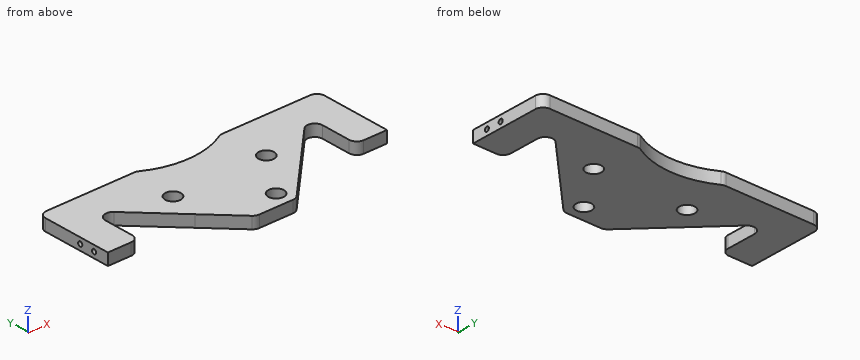
```python
from build123d import *

# Parameters (mm, degrees)
BOSS_EXTRUDE1_DEPTH             = 9.525
F_1_2_0_5_DIAMETER_HOLE1_D      = 12.7
SKETCH7_R                       = 66.675
CUT_EXTRUDE1_DEPTH              = 169.325445566
CUT_EXTRUDE2_DEPTH              = 169.325445566
FILLET1_R                       = 6.35
F_10_24_TAPPED_HOLE1_AT_2_COUNT = 2
F_10_24_TAPPED_HOLE1_AT_2_PITCH = 12.7


with BuildPart() as part:
    # Sketch2 → Boss-Extrude1 (new body)
    with BuildSketch(Plane.XY):
        Polygon((-16.500012242, 33.286517476), (16.500012242, 33.286517476), (42.913494767, 59.7), (114.3, 59.7), (114.3, 123.2), (-114.3, 123.2), (-114.3, 59.7), (-42.913494767, 59.7), align=None)
    extrude(amount=BOSS_EXTRUDE1_DEPTH)

    # 1/2 (0.5) Diameter Hole1 (through all)
    with Locations(Plane.XY.offset(9.525)):
        with Locations((-38.227, 85.227), (38.227, 85.227), (11.2395, 45.986517476)):
            Hole(F_1_2_0_5_DIAMETER_HOLE1_D / 2)

    # Sketch7 → Cut-Extrude1 (cut, through all)
    with BuildSketch(Plane(origin=(0, 0, 0), x_dir=(-1, 0, 0), z_dir=(0, 0, -1))):
        with Locations((0, 180.35)):
            Circle(SKETCH7_R)
    extrude(amount=-CUT_EXTRUDE1_DEPTH, mode=Mode.SUBTRACT)

    # Sketch13 → Cut-Extrude2 (cut, through all)
    with BuildSketch(Plane(origin=(0, 0, 0), x_dir=(-1, 0, 0), z_dir=(0, 0, -1))):
        Polygon((42.913494767, 59.7), (88.9, 105.686505233), (88.9, 59.7), align=None)
        Polygon((-42.913494767, 59.7), (-88.9, 105.686505233), (-88.9, 59.7), align=None)
    extrude(amount=-CUT_EXTRUDE2_DEPTH, mode=Mode.SUBTRACT)

    # Fillet1
    fillet1_edges = [part.edges().sort_by_distance(p)[0] for p in [
        (-114.3, 123.2, 4.7625),
        (114.3, 123.2, 4.7625),
        (16.500012242, 33.286517476, 4.7625),
        (-16.500012242, 33.286517476, 4.7625),
        (-34.342875899, 123.2, 4.7625),
        (34.342875899, 123.2, 4.7625),
        (-88.9, 59.7, 4.7625),
        (-88.9, 105.686505233, 4.7625),
        (88.9, 59.7, 4.7625),
        (88.9, 105.686505233, 4.7625),
    ]]
    fillet(fillet1_edges, radius=FILLET1_R)

    # Sketch12 → #10-24 Tapped Hole1 (revolve, cut)
    with BuildSketch(Plane(origin=(-114.3, 85.1, 4.7625), x_dir=(0, 0, 1), z_dir=(0, 1, 0))):
        Polygon((0, 0), (0, 16.088724014), (1.89865, 14.9479), (1.89865, 0), align=None)
    f_10_24_tapped_hole1 = revolve(axis=Axis((-120.65, 85.1, 4.7625), (1, 0, 0)), mode=Mode.SUBTRACT)

    # #10-24 Tapped Hole1 at 2: #10-24 Tapped Hole1 ×2
    with Locations(*[(0, -i * F_10_24_TAPPED_HOLE1_AT_2_PITCH, 0) for i in range(1, F_10_24_TAPPED_HOLE1_AT_2_COUNT)]):
        add(f_10_24_tapped_hole1, mode=Mode.SUBTRACT)

    # Mirror1: #10-24 Tapped Hole1 across plane
    add(f_10_24_tapped_hole1.mirror(Plane(origin=(0, 0, 0), x_dir=(0, 0, 1), z_dir=(1, 0, 0))), mode=Mode.SUBTRACT)

    # Mirror1 copy 1 sketch → Mirror1 copy 1 (revolve, cut)
    with BuildSketch(Plane(origin=(114.3, 72.4, 4.7625), x_dir=(0, 0, 1), z_dir=(0, 1, 0))):
        Polygon((0, 0), (0, -16.088724014), (1.89865, -14.9479), (1.89865, 0), align=None)
    revolve(axis=Axis((120.65, 72.4, 4.7625), (1, 0, 0)), mode=Mode.SUBTRACT)


solid = part.part
```
CAD build for the part. Positions are in the model's coordinates, mm. Round coordinates to 2 decimals unless told otherwise and drop trailing zeros. Order: outer loops, then holes, each group sorted by start corner. A loop starts at its lowest first (then second) coordinate and runs counter-clockwise, first axis right, second up. Notation, with made-up numbers: (18.5, 28) - (36.5, 28) arc R21 ccw to (36.5, 56) - close; hole circle Ø4 at (29.25, 53.5). An arc over 180 degrees is marked (long way). Use CSV: the item, a comma, the result in double quotes. Start each with the question number.
1) Saw through at A-A (y = 81). List the corners of the cut face in (x, z) (1 decimal), and give its area (3 significant figures).
2) Pin check, flat tips, straight feed: pin 1 Ø3 at (x, z) = (107, 4.5) entering from -Y; pin 2 Ø4 at (x, z) = (-52, 1.5) entering from -Y. Stop position of each tip, or through.
3) Saw through at B-B (x = -91.5). List the corners of the cut face in (y, z) (3 decimals), and give its area (3 significant figures).
4) Wall check: L1, parallel to Z at x = -107, y = 72.4 (3 decimals); L2, parallel to Y at x = 96.5, z = 0.75; L3, parallel to X at y = 86, z = 2. Give the ranges that are in metal, low to high. Write a range as [from, to].
5) Saw through at C-C (x = -66). List the corners of the cut face in (y, z) (1 decimal), and give its area (3 significant figures).
Values follow:
1,outline,"(-114.3, 0) - (-88.9, 0) - (-88.9, 9.5) - (-114.3, 9.5) - close; (-64.2, 0) - (-43, 0) - (-43, 9.5) - (-64.2, 9.5) - close; (-33.5, 0) - (33.5, 0) - (33.5, 9.5) - (-33.5, 9.5) - close; (43, 0) - (64.2, 0) - (64.2, 9.5) - (43, 9.5) - close; (88.9, 0) - (114.3, 0) - (114.3, 9.5) - (88.9, 9.5) - close"
1,area,"1,530 mm2"
2,pin 1,"stops at y = 59.7"
2,pin 2,"stops at y = 66.79"
3,outline,"(60.926, 0) - (123.2, 0) - (123.2, 9.525) - (60.926, 9.525) - close"
3,area,"593 mm2"
4,L1,"z = [0, 2.864], [6.661, 9.525]"
4,L2,"y = [59.7, 123.2]"
4,L3,"x = [-114.3, -88.9], [-69.21, -44.53], [-31.92, 31.92], [44.53, 69.21], [88.9, 114.3]"
5,outline,"(82.8, 0) - (123.2, 0) - (123.2, 9.5) - (82.8, 9.5) - close"
5,area,"385 mm2"
